Geometry check sheet. Reference: the model listing, model coordinates, mm. A direction names the side the tool comes from. Coordinates: 2 decimals unless noted, no trailing zeros. Write each loop counter-clockwise with the first axis right and the second up, starting at its lowest first coordinate (ties: lowest second). Pieces come first, ordered by that corner, then holes. Notation, with made-up numbers: M 56,-26.75 L 82,-26.75 A23 cw 82,3.25 Z; hole C -14,27.25 d7. An arc over 180 degrees is marked long. Answer as a JSON object with one key per item and string values. Group by question number.
```python
from build123d import *

# Parameters (mm, degrees)
SCHIZZO1_W                       = 150
SCHIZZO1_H                       = 80
BASE_FLANGIA1_DEPTH              = 3
BORDO_FLANGIA1_STRIP_W           = 18
BORDO_FLANGIA1_STRIP_H           = 3
BORDO_FLANGIA1_STRIP_CUT_DEPTH   = 150
BORDO_FLANGIA1_STRIP_2_W         = 18
BORDO_FLANGIA1_STRIP_2_H         = 3
BORDO_FLANGIA1_STRIP_CUT_2_DEPTH = 150
BORDO_FLANGIA1_DEPTH             = 150
BORDO_FLANGIA1_BEND_DEPTH        = 150
BORDO_FLANGIA3_STRIP_W           = 13.4732
BORDO_FLANGIA3_STRIP_H           = 3
BORDO_FLANGIA3_STRIP_CUT_DEPTH   = 60
BORDO_FLANGIA3_RELIEF_W          = 14.9732
BORDO_FLANGIA3_RELIEF_H          = 1.5
BORDO_FLANGIA3_RELIEF_CUT_DEPTH  = 3
BORDO_FLANGIA3_DEPTH             = 60
SCHIZZO28_R                      = 2.5
TAGLIO_ESTRUSIONE1_DEPTH         = 3
SCHIZZO30_R                      = 2.5
TAGLIO_ESTRUSIONE2_DEPTH         = 3


# Sheet-metal steps are written as plain solids
with BuildPart() as part:
    # Schizzo1 → Base-Flangia1 (new body)
    with BuildSketch(Plane.XY):
        Rectangle(SCHIZZO1_W, SCHIZZO1_H)
    extrude(amount=-BASE_FLANGIA1_DEPTH)

    # Bordo-Flangia1 strip (across the edge) → Bordo-Flangia1 strip cut (cut)
    with BuildSketch(Plane(origin=(-75, 40, -3), x_dir=(0, -1, 0), z_dir=(1, 0, 0))):
        with Locations((-3, -1.5)):
            Rectangle(BORDO_FLANGIA1_STRIP_W, BORDO_FLANGIA1_STRIP_H)
    extrude(amount=BORDO_FLANGIA1_STRIP_CUT_DEPTH, mode=Mode.SUBTRACT)

    # Bordo-Flangia1 strip 2 (across the edge) → Bordo-Flangia1 strip cut 2 (cut)
    with BuildSketch(Plane(origin=(75, -40, -3), x_dir=(0, 1, 0), z_dir=(-1, 0, 0))):
        with Locations((-3, -1.5)):
            Rectangle(BORDO_FLANGIA1_STRIP_2_W, BORDO_FLANGIA1_STRIP_2_H)
    extrude(amount=BORDO_FLANGIA1_STRIP_CUT_2_DEPTH, mode=Mode.SUBTRACT)

    # Bordo-Flangia1 section (across the edge) → Bordo-Flangia1 (add)
    with BuildSketch(Plane(origin=(-75, 40, -3), x_dir=(0, -1, 0), z_dir=(1, 0, 0))):
        with BuildLine():
            Line((0, 3), (0, 30))
            Line((0, 30), (3, 30))
            Line((3, 30), (3, 3))
            ThreePointArc((3, 3), (3.878679656, 0.878679656), (6, 0))
            Line((6, 0), (6, -3))
            ThreePointArc((6, -3), (1.757359313, -1.242640687), (0, 3))
        make_face()
    extrude(amount=BORDO_FLANGIA1_DEPTH)

    # Bordo-Flangia1 section 2 (across the edge) → Bordo-Flangia1 bend (add)
    with BuildSketch(Plane(origin=(75, -40, -3), x_dir=(0, 1, 0), z_dir=(-1, 0, 0))):
        with BuildLine():
            Line((0, 3), (0, 30))
            Line((0, 30), (3, 30))
            Line((3, 30), (3, 3))
            ThreePointArc((3, 3), (3.878679656, 0.878679656), (6, 0))
            Line((6, 0), (6, -3))
            ThreePointArc((6, -3), (1.757359313, -1.242640687), (0, 3))
        make_face()
    extrude(amount=BORDO_FLANGIA1_BEND_DEPTH)

    # Bordo-Flangia3 strip (across the edge) → Bordo-Flangia3 strip cut (cut)
    with BuildSketch(Plane(origin=(-75, 30, 0), x_dir=(1, 0, 0), z_dir=(0, -1, 0))):
        with Locations((-3, -1.5)):
            Rectangle(BORDO_FLANGIA3_STRIP_W, BORDO_FLANGIA3_STRIP_H)
    extrude(amount=BORDO_FLANGIA3_STRIP_CUT_DEPTH, mode=Mode.SUBTRACT)

    # Bordo-Flangia3 relief (on the sheet) → Bordo-Flangia3 relief cut (cut)
    with BuildSketch(Plane(origin=(-71.2634, 30, 0), x_dir=(1, 0, 0), z_dir=(0, 0, 1))):
        with Locations((-5.9866, 0.75)):
            Rectangle(BORDO_FLANGIA3_RELIEF_W, BORDO_FLANGIA3_RELIEF_H)
        with Locations((-5.9866, -60.75)):
            Rectangle(BORDO_FLANGIA3_RELIEF_W, BORDO_FLANGIA3_RELIEF_H)
    extrude(amount=-BORDO_FLANGIA3_RELIEF_CUT_DEPTH, mode=Mode.SUBTRACT)

    # Bordo-Flangia3 section (across the edge) → Bordo-Flangia3 (add)
    with BuildSketch(Plane(origin=(-75, 30, 0), x_dir=(1, 0, 0), z_dir=(0, -1, 0))):
        with BuildLine():
            Line((0, 0.7366), (0, 60))
            Line((0, 60), (3, 60))
            Line((3, 60), (3, 0.7366))
            ThreePointArc((3, 0.7366), (3.215745145, 0.215745145), (3.7366, 0))
            Line((3.7366, 0), (3.7366, -3))
            ThreePointArc((3.7366, -3), (1.094424801, -1.905575199), (0, 0.7366))
        make_face()
    extrude(amount=BORDO_FLANGIA3_DEPTH)

    # Schizzo28 → Taglio-Estrusione1 (cut)
    with BuildSketch(Plane(origin=(-72, 0, 0), x_dir=(0, 0, -1), z_dir=(1, 0, 0))):
        with BuildLine():
            Line((-60, 30), (-60, 10))
            ThreePointArc((-60, 10), (-54.142135624, 24.142135624), (-40, 30))
            Line((-40, 30), (-60, 30))
        make_face()
        with BuildLine():
            ThreePointArc((-40, -30), (-54.142135624, -24.142135624), (-60, -10))
            Line((-60, -10), (-60, -30))
            Line((-60, -30), (-40, -30))
        make_face()
        with BuildLine():
            Line((-34.898979486, -11.5), (-25.101020514, -11.5))
            ThreePointArc((-25.101020514, -11.5), (-17.5, 0), (-25.101020514, 11.5))
            Line((-25.101020514, 11.5), (-34.898979486, 11.5))
            ThreePointArc((-34.898979486, 11.5), (-42.5, 0), (-34.898979486, -11.5))
        make_face()
        with Locations((-42.374368671, 12.374368671)):
            Circle(SCHIZZO28_R)
        with Locations((-17.625631329, 12.374368671)):
            Circle(SCHIZZO28_R)
        with Locations((-17.625631329, -12.374368671)):
            Circle(SCHIZZO28_R)
        with Locations((-42.374368671, -12.374368671)):
            Circle(SCHIZZO28_R)
    extrude(amount=-TAGLIO_ESTRUSIONE1_DEPTH, mode=Mode.SUBTRACT)

    # Schizzo30 → Taglio-Estrusione2 (cut)
    with BuildSketch(Plane.XY):
        with Locations((-24.5, 0)):
            Circle(SCHIZZO30_R)
        with Locations((-4.5, 0)):
            Circle(SCHIZZO30_R)
    extrude(amount=-TAGLIO_ESTRUSIONE2_DEPTH, mode=Mode.SUBTRACT)


solid = part.part
```
1) Go/stop test with flat-tipped pins: pin 1 Ø2 at (y, z) = (-11.5, 40) entering from +X; pin 2 Ø3.5 at (x, z) = (-72.5, -1.5) entering from +Y; pin 3 Ø1.5 at (x, z) = (-74, 32) entering from -Y. Record where each tip stops, or that it passes through.
2) Draft check along Y on faces 5 (the flat face through (-75, -38, -13)), 6 (the cylindrical face through (-1.05, 38.196, -1.711)), 7 (the cylindrical face through (1.05, -36.14, -3.9)). Enter one of: +Y half, -Y half, draft (parallel to the pull), parting line (faces both ways), or undercut.
3) Section check C-C (y = 0). Record the cut outline in (x, z).
4) Section check A-A (z = 28.5). Record the cut outline in (x, y), then the cut area to 3 significant figures.
5) Material ranges on probe 1 along Y at (x, z) = (-65.5, -9.5); probe 2 along Z at (x, y) = (-69, -25); probe 3 along X at (y, z) = (-17, 50.5), recorded low to high. Write a range as [from, to].
6) Section check B-B (x = -24.5). Record the cut outline in (y, z), then the cut area to 3 significant figures.
7) Section check D-D (y = 22). Record the cut outline in (x, z), then the cut area to 3 significant figures.
8) Set-up check for faces 1 (the flat face through (-72, -13, 31)), 2 (the cylindrical face through (-1.05, 36.14, -3.9)), 3 (the flat face through (-72, -31.5, -1)), 4 (the cylindrical face through (-73.88, 0.42, -1.93)): record each of +Z, -Z, +X, -X, +Y, -Y from which the full face is reachable in a straight line by a thin tool's end or side.
Entries:
{
 "1": {"pin 1": "x = -72", "pin 2": "y = 39.33", "pin 3": "y = -30"},
 "2": {"face 5": "draft", "face 6": "+Y half", "face 7": "undercut"},
 "3": {"outline": "M -75,0.74 A3.74 ccw -71.26,-3 L -27,-3 L -27,0 L -71.26,0 A0.74 cw -72,0.74 L -72,17.5 L -75,17.5 Z; M -75,42.5 L -72,42.5 L -72,60 L -75,60 Z; M -22,-3 L -7,-3 L -7,0 L -22,0 Z; M -2,-3 L 75,-3 L 75,0 L -2,0 Z"},
 "4": {"outline": "M -75,-30 L -72,-30 L -72,-11.5 L -75,-11.5 Z; M -75,11.5 L -72,11.5 L -72,30 L -75,30 Z", "area": "111 mm^2"},
 "5": {"probe 1": "[-40, -37], [37, 40]", "probe 2": "[-3, 0]", "probe 3": "[-75, -72]"},
 "6": {"outline": "M -40,-33 L -37,-33 L -37,-6 A3 cw -34,-3 L -2.5,-3 L -2.5,0 L -34,0 A6 ccw -40,-6 Z; M 2.5,-3 L 34,-3 A3 cw 37,-6 L 37,-33 L 40,-33 L 40,-6 A6 ccw 34,0 L 2.5,0 Z", "area": "393 mm^2"},
 "7": {"outline": "M -75,0.74 A3.74 ccw -71.26,-3 L 75,-3 L 75,0 L -71.26,0 A0.74 cw -72,0.74 L -72,56 L -75,56 Z", "area": "615 mm^2"},
 "8": {"face 1": "+Z, +X, +Y, -Y", "face 2": "-Z, +X, -X", "face 3": "+Z, -Z, -X", "face 4": "-Z, -X"}
}
